The figure shows three views and two pictorial views of one solid part (mm, origin at its lowest corner). Answer the questions. A direction names the side the tool comes from. Coordinates: 2 decimals unless noted, no trailing zeros. Order: outer loops, then holes, each group sorted by start corner. A loop starts at its lowest first (then second) coordinate and runs counter-clockwise, first axis right, second up. Notation, with made-up numbers: M 62.5,74 L 86.5,74 A28 ccw 86.5,101 Z; hole C 34.25,-2.75 d3. An arc over 180 degrees is marked long. Answer in a Markdown table with one row per item. Add a question column.
Item 1: The part is cut by section A-A (x = 26). Write down the section's boundary in (y, z), then the cut area to 3 significant figures.
Item 2: Consider line 1 (X direction, y = 33, z = 13.5) (1 decimal); line 2 (Z direction, x = 55, y = 40); line 3 (X direction, y = 40, z = 17.5) (1 decimal). Determine where each line is inside the solid, lowest interval first. Write a range as from..to.
Item 3: Which of the six approach directions +Z, -Z, +X, -X, +Y, -Y give full straight-line access (tool end or side, diameter ignored) to the marked faces 1 and 2?
Item 4: The mould has two halves that part along X. Classify the marked faces 3 and 4: released by +X, released by -X, zero draft, split by the parting line, or undercut.
Item 5: The part is cut by section B-B (z = 3.75). Write down the section's boundary in (x, y), then the cut area to 3 significant figures.
Item 6: The part is cut by section C-C (y = 12). Write down the section's boundary in (x, z).
Item 7: Flat-ended cylindrical pins translate along their axes: pin 1 Ø5 at (x, y) = (51.5, 22.5) entering from +Z; pin 2 Ø5.5 at (x, y) = (55.245, 3.175) entering from -Z; pin 3 Ø10 at (y, z) = (17.5, 8.5) entering from -X; pin 4 Ø8 at (x, z) = (39.5, 19.5) entering from +Y. Find the tip coordinate at first contact, or state that the pin passes through.
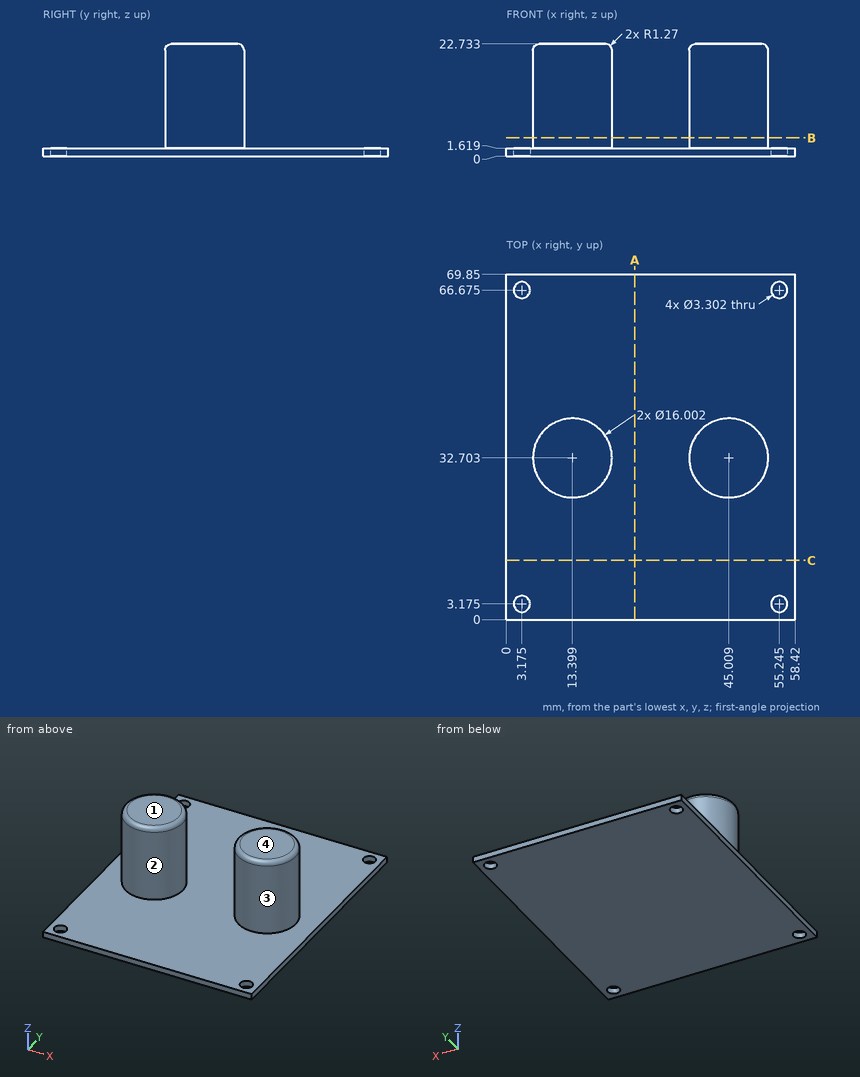
Reply:
| question | item | result |
|---|---|---|
| 1 | outline | M 0,0 L 69.85,0 L 69.85,1.62 L 0,1.62 Z |
| 1 | area | 113 mm2 |
| 2 | line 1 | x = 5.4..21.4, 37..53 |
| 2 | line 2 | z = 0..1.62 |
| 2 | line 3 | x = 10.1..16.7, 41.7..48.3 |
| 3 | face 1 | +Z, +X, -X, +Y, -Y |
| 3 | face 2 | +Z |
| 4 | face 3 | undercut |
| 4 | face 4 | zero draft |
| 5 | outline | C 13.4,32.7 d16; C 45.01,32.7 d16 |
| 5 | area | 402 mm2 |
| 6 | outline | M 0,0 L 58.42,0 L 58.42,1.62 L 0,1.62 Z |
| 7 | pin 1 | stops at z = 1.62 |
| 7 | pin 2 | stops at z = 0 |
| 7 | pin 3 | passes through |
| 7 | pin 4 | stops at y = 40.56 |
